Part model, mm, in its own coordinate system. A direction names the side the tool comes from. Round coordinates to 2 decimals unless told otherwise and drop trailing zeros. Write each loop counter-clockwise with the first axis right and the second up, starting at its lowest first coordinate (ties: lowest second). Pieces come first, ordered by that corner, then holes.
Solid Edge part; units mm, degrees
sketch "Sketch1" plane through (0, 0, 0) normal (0, -1, 0) x (1, 0, 0)
  circle A0 centre (0, 0) radius 4.5
  circle A1 centre (-5.5, 20) radius 1.6
  circle A2 centre (5.5, 20) radius 1.6
  circle A3 centre (-5.5, -20) radius 1.6
  circle A4 centre (5.5, -20) radius 1.6
  line L0 (-9, -24) -> (9, -24)
  line L1 (9, -24) -> (9, 24)
  line L2 (9, 24) -> (-9, 24)
  line L3 (-9, 24) -> (-9, -24)
  dimension "D1" = 9
  dimension "D2" = 9
extrude "Protrusion1" add sketch "Sketch1" along normal blind 6
sketch "Sketch2" plane through (0, -6, 0) normal (0, -1, 0) x (1, 0, 0)
  circle A0 centre (0, 0) radius 6.5
extrude "ExtrudedCutout_1" cut sketch "Sketch2" against normal blind 2.5
hole "Hole_5" at (-5, 0, -7.5) direction (0, -1, 0) diameter 2.459 end up to next
hole "Hole1" at (-5, 0, 7.5) direction (0, -1, 0) diameter 2.459 end up to next
hole "Hole2" at (5, 0, 7.5) direction (0, -1, 0) diameter 2.459 end up to next
hole "Hole3" at (5, 0, -7.5) direction (0, -1, 0) diameter 2.459 end up to next
sketch "Sketch3" plane through (0, 0, 0) normal (0, 1, 0) x (-1, 0, 0)
  circle A0 centre (-5.5, -20) radius 2.9
  circle A1 centre (5.5, -20) radius 2.9
  circle A2 centre (5.5, 20) radius 2.9
  circle A3 centre (-5.5, 20) radius 2.9
extrude "ExtrudedCutout_2" cut sketch "Sketch3" against normal blind 3
Q1. Drop flat-ended pins along their axis: P1, Ø4.5, axis at x = -4.5, z = 20, coming from the +Y side; P2, Ø3.5, axis at x = -5.5, z = 20, coming from the +Y side; P3, Ø2, axis at x = 5, z = 7.5, coming from the +Y side. Give the stop position or say it passes through.
Q2. Two-plate mould, pull along X, no slides. Class faces 4 (the flat face through (0, 0, 6)), 5 (the cylindrical face through (-6.09, -2.96, -6.93)), 6 (the flat face through (9, -3, 0)): released by +X, released by -X, zero draft, split by the parting line, or undercut.
Q3. Tool access for faces 1 (the flat face through (4.42, -3.5, 1.54)), 2 (the cylindrical face through (-3.199, -1.479, -21.765)), 3 (the cylindrical face through (3.91, -2.96, -6.93)): list every direction of +Z, -Z, +X, -X, +Y, -Y with a clear straight run to the whole face (end or side of a thin tool).
Q4. Saw through at B-B, the plane z = -20. Write the cut outline in (x, y).
Q5. Saw through at C-C, the plane y = -4.9. Give the number of separate pieces and of enclosed holes in the cut face, and give its area (3 significant figures).
Q6. Saw through at A-A, the plane x = 0. Write the cut outline in (y, z), and give its area (3 significant figures).
Q7. Wall check: line 1 (X direction, y = -4.15, z = 20); line 2 (X direction, y = -4.55, z = -7.5); line 3 (Z direction, x = 5.5, y = -5.15). Give the ranges that are in metal, low to high.
Q8. Saw through at D-D, the plane z = 0. Write the cut outline in (x, y), and give its area (3 significant figures).
Computed:
1. P1: stops at y = 0
1. P2: stops at y = -3
1. P3: passes through
2. face 4: zero draft
2. face 5: undercut
2. face 6: released by +X
3. face 1: -Y
3. face 2: +Y
3. face 3: +Y, -Y
4. outline: (-9, -6) - (-7.1, -6) - (-7.1, -3) - (-8.4, -3) - (-8.4, 0) - (-9, 0) - close; (-3.9, -6) - (3.9, -6) - (3.9, -3) - (2.6, -3) - (2.6, 0) - (-2.6, 0) - (-2.6, -3) - (-3.9, -3) - close; (7.1, -6) - (9, -6) - (9, 0) - (8.4, 0) - (8.4, -3) - (7.1, -3) - close
5. separate pieces: 1
5. enclosed holes: 9
5. area: 680 mm2
6. outline: (-6, -24) - (0, -24) - (0, -4.5) - (-3.5, -4.5) - (-3.5, -6.5) - (-6, -6.5) - close; (-6, 6.5) - (-3.5, 6.5) - (-3.5, 4.5) - (0, 4.5) - (0, 24) - (-6, 24) - close
6. area: 224 mm2
7. line 1: x = -9 to -7.1, -3.9 to 3.9, 7.1 to 9
7. line 2: x = -9 to -6.23, -3.77 to 3.77, 6.23 to 9
7. line 3: z = -24 to -21.6, -18.4 to -8.62, -6.38 to -3.46, 3.46 to 6.38, 8.62 to 18.4, 21.6 to 24
8. outline: (-9, -6) - (-6.5, -6) - (-6.5, -3.5) - (-4.5, -3.5) - (-4.5, 0) - (-9, 0) - close; (4.5, -3.5) - (6.5, -3.5) - (6.5, -6) - (9, -6) - (9, 0) - (4.5, 0) - close
8. area: 44.0 mm2
